from build123d import *

# Parameters (mm, degrees)
SKETCH_1_W               = 190
SKETCH_1_H               = 40
EXTRUDE_1_DEPTH          = 1500
SKETCH_4_W               = 18.18
SKETCH_4_H               = 60.16888381
CUT_EXTRUDE_1_DEPTH      = 1500
MIRROR_2_COPY_1_SKETCH_W = 18.18
MIRROR_2_COPY_1_SKETCH_H = 60.16888381
MIRROR_2_COPY_1_DEPTH    = 1500


with BuildPart() as part:
    # Sketch 1 → Extrude 1 (new body)
    with BuildSketch(Plane.XY):
        with Locations((95, -20)):
            Rectangle(SKETCH_1_W, SKETCH_1_H)
    extrude(amount=-EXTRUDE_1_DEPTH)

    # Sketch 4 → Cut-Extrude 1 (cut, along a direction that is not the sketch's normal)
    with BuildSketch(Plane(origin=(0, 0, 0), x_dir=(1, 0, 0), z_dir=(0, 1, 0))):
        with Locations((127.243345581, 196.784441905)):
            Rectangle(SKETCH_4_W, SKETCH_4_H)
    cut_extrude_1 = extrude(amount=-CUT_EXTRUDE_1_DEPTH, dir=(-0.18489307241243372, 0.9800002075530074, -0.07358087366940451), mode=Mode.SUBTRACT)

    # Mirror 1: Cut-Extrude 1 across plane
    add(cut_extrude_1.mirror(Plane.XY.offset(-750)), mode=Mode.SUBTRACT)

    # Mirror 2: Cut-Extrude 1 across plane
    add(cut_extrude_1.mirror(Plane(origin=(95, 0, 0), x_dir=(0, 0, 1), z_dir=(1, 0, 0))), mode=Mode.SUBTRACT)

    # Mirror 2 copy 1 sketch → Mirror 2 copy 1 (cut, along a direction that is not the sketch's normal)
    with BuildSketch(Plane(origin=(190, 0, -1500), x_dir=(-1, 0, 0), z_dir=(0, 1, 0))):
        with Locations((127.243345581, 196.784441905)):
            Rectangle(MIRROR_2_COPY_1_SKETCH_W, MIRROR_2_COPY_1_SKETCH_H)
    extrude(amount=-MIRROR_2_COPY_1_DEPTH, dir=(0.18489307241243372, 0.9800002075530074, 0.07358087366940451), mode=Mode.SUBTRACT)


solid = part.part
The listing builds one solid part. Answer for the finished solid, in the listing's coordinates (mm). A direction names the side the tool comes from. Coordinates: 2 decimals unless noted, no trailing zeros. Loops run counter-clockwise (first coordinate to the right, second up) from the corner with the lowest first, then second, coordinate; pieces in that order, holes last.
1) Find section A-A on z = -183.5. Write down the section's boundary in (x, y), then the cut area to 3 significant figures.
2) Find the intervals of material crossed by L1, parallel to Z at x = 132, y = -21.5; L2, parallel to Z at x = 121, y = -10, in increasing order.
3) Determine the mould class of faces 3 (the face through (94, -20, 0)), 4 (the face through (130.84, -19.72, -1274.61)), 5 (the face through (0, -20, -740)), 6 (the face through (140.054, -19.72, -194.841)) for opening direction Z: pulls with the +Z half, pulls with the -Z half, needs draft (parallel to the pull), parting line crosses it, or undercut.
4) A tool of negligible diameter and unlimited length cuts with its end or side. For faces 1 (the face through (130.84, -19.72, -1334.78)), 2 (the face through (94, 0, -740)), from which of +Z, -Z, +X, -X, +Y, -Y can it reach the whole face along a straight path? Write none if from no direction.
5) Find section B-B on y = -18. Write down the section's boundary in (x, z), then the cut area to 3 significant figures.
Values:
1. outline: (0, -40) - (46.12, -40) - (53.67, 0) - (0, 0) - close; (64.3, -40) - (125.7, -40) - (118.15, 0) - (71.85, 0) - close; (136.33, 0) - (143.88, -40) - (190, -40) - (190, 0) - close
1. area: 6,150 mm2
2. L1: z = -1500 to -1334.91, -1274.75 to -225.25, -165.09 to 0
2. L2: z = -1500 to -1334.05, -1273.88 to -226.12, -165.95 to 0
3. face 3: pulls with the +Z half
3. face 4: undercut
3. face 5: needs draft
3. face 6: undercut
4. face 1: none
4. face 2: +Z, -Z, +X, -X, +Y
5. outline: (0, -1500) - (190, -1500) - (190, 0) - (0, 0) - close; hole (50.27, -1334.65) - (68.45, -1334.65) - (68.45, -1274.48) - (50.27, -1274.48) - close; hole (50.27, -225.52) - (68.45, -225.52) - (68.45, -165.35) - (50.27, -165.35) - close; hole (121.55, -1334.65) - (139.73, -1334.65) - (139.73, -1274.48) - (121.55, -1274.48) - close; hole (121.55, -225.52) - (139.73, -225.52) - (139.73, -165.35) - (121.55, -165.35) - close
5. area: 281,000 mm2
